Here's how the part is built. I have some questions about the finished solid (model axes, mm). A direction names the side the tool comes from. Coordinates: 2 decimals unless noted, no trailing zeros. Write each loop counter-clockwise with the first axis right and the second up, starting at its lowest first coordinate (ties: lowest second). Pieces come first, ordered by that corner, then holes. Notation, with made-up numbers: (36, 31) -> (71, 31) arc R14 cw to (71, 36) -> close; hole circle Ø9 at (-22, 35.5). An arc over 180 degrees is marked (long way). Put each result on its own line as item: value. Start each with the question number.
Item 1: For pin 1 (1.2 mm diameter, centred on x = -6.5, z = 2, fed in from -Y); pin 2 (1.5 mm diameter, centred on y = -12, z = 2, fed in from +X); pin 3 (1.5 mm diameter, centred on y = -11, z = 1, fed in from -X), each with a flat end and sliding along its axis, tell me the tip position at first contact or that it passes through.
Item 2: I want a section at B-B, the plane z = 2.6. List the corners of the cut face in (x, y) for me.
Item 3: I want a section at C-C, the plane y = 0.5. List the corners of the cut face in (x, z) for me, then the cut area to 3 significant figures.
Item 4: I want a section at A-A, the plane x = 0.5. List the corners of the cut face in (y, z) for me, then the cut area to 3 significant figures.
Item 5: I need wall thicknesses on line 1 (X direction, y = -6.5, z = 2.8); line 2 (X direction, y = -10.5, z = 0.5); line 3 (Y direction, x = 3, z = 0.3). Which ranges of each line are inside material? Lowest first, please. Write a range as [from, to].
Item 6: If we mould it in two halves opening along Y, with no side actions, what happens to faces 1 (the face through (-0.27, -1.22, 1.48)), 2 (the face through (-5.859, 2.797, 1.521)), 3 (the face through (4, 0, 1)), 4 (the face through (-7, -5, 1))? For each: released by +Y, released by -Y, zero draft, split by the parting line, or undercut.
Item 7: I want a section at D-D, the plane y = -10.75. List the corners of the cut face in (x, z) for me.
Item 8: On a 3-axis mill with a long thin cutter (end or side, diameter ignored), from which of +Z, -Z, +X, -X, +Y, -Y can I reach the whole of each face in a straight line? I mean faces 5 (the face through (-5.5, -11, 1)), 6 (the face through (-3, -2, 0)), 7 (the face through (-1, -10, 1)). Say none if no direction works.
from build123d import *

# Parameters (mm, degrees)
SKETCH1_R           = 1.25
BOSS_EXTRUDE1_DEPTH = 3
FILLET1_R           = 4


with BuildPart() as part:
    # Sketch1 → Boss-Extrude1 (new body)
    with BuildSketch(Plane.XY):
        with BuildLine():
            Line((-7, 4), (-7, -10))
            Line((-7, -10), (-5.5, -10))
            Line((-5.5, -10), (-5.5, -13))
            Line((-5.5, -13), (-1.5, -13))
            Line((-1.5, -13), (-1.5, -10))
            Line((-1.5, -10), (0, -10))
            Line((0, -10), (0, -4))
            ThreePointArc((0, -4), (4, 0), (0, 4))
            Line((0, 4), (-7, 4))
        make_face()
        Circle(SKETCH1_R, mode=Mode.SUBTRACT)
    extrude(amount=BOSS_EXTRUDE1_DEPTH)

    # Fillet1
    fillet1_edges = [part.edges().sort_by_distance(p)[0] for p in [
        (-7, 4, 1.5),
    ]]
    fillet(fillet1_edges, radius=FILLET1_R)


solid = part.part
Calculated:
1. pin 1: stops at y = -10
1. pin 2: stops at x = -1.5
1. pin 3: stops at x = -5.5
2. outline: (-7, -10) -> (-5.5, -10) -> (-5.5, -13) -> (-1.5, -13) -> (-1.5, -10) -> (0, -10) -> (0, -4) arc R4 ccw to (0, 4) -> (-3, 4) arc R4 ccw to (-7, 0) -> close; hole circle Ø2.5 at (0, 0)
3. outline: (-6.97, 0) -> (-1.15, 0) -> (-1.15, 3) -> (-6.97, 3) -> close; (1.15, 0) -> (3.97, 0) -> (3.97, 3) -> (1.15, 3) -> close
3. area: 25.9 mm2
4. outline: (-3.97, 0) -> (-1.15, 0) -> (-1.15, 3) -> (-3.97, 3) -> close; (1.15, 0) -> (3.97, 0) -> (3.97, 3) -> (1.15, 3) -> close
4. area: 16.9 mm2
5. line 1: x = [-7, 0]
5. line 2: x = [-5.5, -1.5]
5. line 3: y = [-2.65, 2.65]
6. face 1: undercut
6. face 2: released by +Y
6. face 3: split by the parting line
6. face 4: zero draft
7. outline: (-5.5, 0) -> (-1.5, 0) -> (-1.5, 3) -> (-5.5, 3) -> close
8. face 5: +Z, -Z, -X, -Y
8. face 6: -Z, +X, -X, +Y, -Y
8. face 7: +Z, -Z, +X, -Y
